Geometry check sheet. Reference: the model listing, model coordinates, mm. Face numbers are marked on the shaded views. A direction names the side the tool comes from. Coordinates: 2 decimals unless noted, no trailing zeros. Order: outer loops, then holes, each group sorted by start corner. A loop starts at its lowest first (then second) coordinate and runs counter-clockwise, first axis right, second up. Notation, with made-up numbers: (40.25, -29.75) - (75.25, -29.75) arc R18 ccw to (75.25, -18.75) - close; hole circle Ø7 at (86.25, 82). An arc over 180 degrees is marked (long way). Return JSON: item names as keys, results as strings. Group by question number.
Item 1: Draft check along Y on the marked faces 3, 4 and 5. Enter one of: pulls with the +Y half, pulls with the -Y half, needs draft (parallel to the pull), parting line crosses it, or undercut.
Item 2: Section check A-A on z = 0. Enter the section's corners in (x, y).
Item 3: Section check B-B on x = 4.5. Enter the section's corners in (y, z).
Item 4: Gauge pin test, flat ends, axial feed: pin 1 (1.5 mm diameter, centred on x = -1.5, z = -17, fed in from +Y); pin 2 (2 mm diameter, centred on x = 1, z = 9.5, fed in from +Y); pin 3 (4.5 mm diameter, centred on y = -20.25, z = 0, fed in from -X); pin 4 (1 mm diameter, centred on x = 2.5, y = -7.5, fed in from +Z). Record the tip position at first contact, or that the pin passes through.
Item 5: Scan lines: probe 1 along Z at (x, y) = (-5.75, -20); probe 2 along Y at (x, z) = (6.55, 0); probe 3 along Y at (x, z) = (-0.75, -6). Record each from-to range of solid material in increasing order.
Item 6: Section check C-C on x = -0.5. Enter the section's corners in (y, z), then the cut area to 3 significant figures.
Item 7: Tool access check on the marked faces 1 and 2. Record the directions out of +Z, -Z, +X, -X, +Y, -Y that give a thin tool (end or side, any length) a straight path to the whole face; none if there is none.
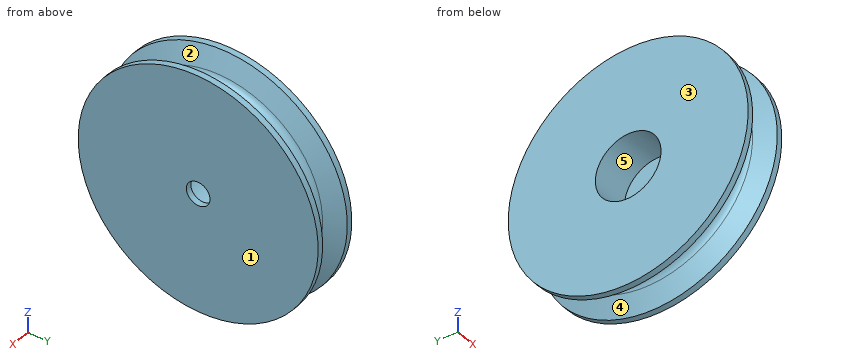
from build123d import *

# Parameters (mm, degrees)
CROQUIS2_R            = 3.95
CORTAR_EXTRUIR1_DEPTH = 62
CROQUIS3_R            = 10.95
CORTAR_EXTRUIR2_DEPTH = 13


with BuildPart() as part:
    # Croquis1 → Revolución1 (revolve)
    with BuildSketch(Plane.XY, mode=Mode.PRIVATE) as revoluci_n1_sk:
        with BuildLine():
            Line((5.952239129, 19.74561549), (2.952239129, 13.74561549))
            ThreePointArc((2.952239129, 13.74561549), (0.452239129, 12.151246549), (-2.047760871, 13.74561549))
            Line((-2.047760871, 13.74561549), (-5.047760871, 19.74561549))
            Line((-5.047760871, 19.74561549), (-7.047760871, 19.74561549))
            Line((-7.047760871, 19.74561549), (-7.047760871, -20.25438451))
            Line((-7.047760871, -20.25438451), (7.952239129, -20.25438451))
            Line((7.952239129, -20.25438451), (7.952239129, 19.74561549))
            Line((7.952239129, 19.74561549), (5.952239129, 19.74561549))
        make_face()
    revolve(revoluci_n1_sk.sketch.rotate(Axis((-20.844407183, -20.25438451, 0), (1, 0, 0)), 90), axis=Axis((-20.844407183, -20.25438451, 0), (1, 0, 0)))

    # Croquis2 → Cortar-Extruir1 (cut)
    with BuildSketch(Plane.ZY.offset(7.047760871)):
        with Locations((0, -20.25438451)):
            Circle(CROQUIS2_R)
    extrude(amount=-CORTAR_EXTRUIR1_DEPTH, mode=Mode.SUBTRACT)

    # Croquis3 → Cortar-Extruir2 (cut)
    with BuildSketch(Plane.ZY.offset(7.047760871)):
        with Locations((0, -20.25438451)):
            Circle(CROQUIS3_R)
    extrude(amount=-CORTAR_EXTRUIR2_DEPTH, mode=Mode.SUBTRACT)


solid = part.part
Computed:
{
 "1": {"face 3": "needs draft", "face 4": "parting line crosses it", "face 5": "undercut"},
 "2": {"outline": "(-7.05, -60.25) - (-5.05, -60.25) - (-2.05, -54.25) arc R2.76 cw to (2.95, -54.25) - (5.95, -60.25) - (7.95, -60.25) - (7.95, -24.2) - (5.95, -24.2) - (5.95, -31.2) - (-7.05, -31.2) - close; (-7.05, -9.3) - (5.95, -9.3) - (5.95, -16.3) - (7.95, -16.3) - (7.95, 19.75) - (5.95, 19.75) - (2.95, 13.75) arc R2.76 cw to (-2.05, 13.75) - (-5.05, 19.75) - (-7.05, 19.75) - close"},
 "3": {"outline": "circle Ø74.19 at (-20.25, 0); hole circle Ø21.9 at (-20.25, 0)"},
 "4": {"pin 1": "stops at y = 9.71", "pin 2": "stops at y = 11.29", "pin 3": "passes through", "pin 4": "stops at z = 31.64"},
 "5": {"probe 1": "z = -40 to -10.95, 10.95 to 40", "probe 2": "y = -60.25 to -24.2, -16.3 to 19.75", "probe 3": "y = -52.38 to -29.41, -11.09 to 11.87"},
 "6": {"outline": "circle Ø65.15 at (-20.25, 0); hole circle Ø21.9 at (-20.25, 0)", "area": "2,960 mm²"},
 "7": {"face 1": "+Z, -Z, +X, +Y, -Y", "face 2": "none"}
}
